```python
from build123d import *

# Parameters (mm, degrees)
SKETCH2_R               = 0.5
CUT_EXTRUDE1_DEPTH      = 4
CUT_EXTRUDE1_DEPTH_BACK = 4


with BuildPart() as part:
    # Sketch1 → Revolve1 (revolve)
    with BuildSketch(Plane.XY):
        with BuildLine():
            Line((0, 0), (0, 1.5))
            Line((0, 1.5), (0.5, 2))
            Line((0.5, 2), (39, 2))
            Line((39, 2), (39, 3))
            ThreePointArc((39, 3), (41.121320344, 2.121320344), (42, 0))
            Line((42, 0), (0, 0))
        make_face()
    revolve(axis=Axis((0, 0, 0), (1, 0, 0)))

    # Sketch2 → Cut-Extrude1 (cut, two sides)
    with BuildSketch(Plane.XY) as cut_extrude1_sk:
        with Locations((2, 0)):
            Circle(SKETCH2_R)
    extrude(amount=CUT_EXTRUDE1_DEPTH, mode=Mode.SUBTRACT)
    extrude(cut_extrude1_sk.sketch, amount=-CUT_EXTRUDE1_DEPTH_BACK, mode=Mode.SUBTRACT)


solid = part.part
```
Model file for the job. Use its own axes, mm. A direction names the side the tool comes from. Coordinates: 2 decimals unless noted, no trailing zeros. Loops run counter-clockwise (first coordinate to the right, second up) from the corner with the lowest first, then second, coordinate; pieces in that order, holes last. Notation, with made-up numbers: M 59.25,13 L 71.25,13 A20 ccw 71.25,22 Z; hole C 53,79 d7. An arc over 180 degrees is marked long. Use CSV: the item, a comma, the result in double quotes. Start each with the question number.
1. Band-saw the part on B-B, the plane x = 24. List the corners of the cut face in (y, z), then the cut area to 3 significant figures.
2. Band-saw the part on A-A, the plane y = 0. List the corners of the cut face in (x, z), then the cut area to 3 significant figures.
3. Flat gauge pins, fed straight in: pin 1 (1.5 mm diameter, centred on x = 27, z = -0.5, fed in from -Y); pin 2 (1 mm diameter, centred on x = 18, z = -1, fed in from -Y); pin 3 (1 mm diameter, centred on x = 17, y = 2, fed in from +Z). Where does each tip first touch, or does it go through?
4. Band-saw the part on D-D, the plane y = -2.6. List the corners of the cut face in (x, z), then the cut area to 3 significant figures.
5. Band-saw the part on C-C, the plane x = 2. List the corners of the cut face in (y, z).
6. Tool access for faces 1 (the cylindrical face through (20, 0, -2)), 2 (the flat face through (0, 0, 0)): list every direction of +Z, -Z, +X, -X, +Y, -Y with a clear straight run to the whole face (end or side of a thin tool).
7. Probe probe 1 along Y at (x, z) = (2, 0.6); probe 2 along X at (y, z) = (0, 0.45); probe 3 along Y at (x, z) = (2, -1.4). List the from-to ranges inside material, lowest first. Write a range as [from, to].
Entries:
1,outline,"C 0,0 d4"
1,area,"12.6 mm2"
2,outline,"M 0,-1.5 L 0.5,-2 L 1.5,-2 L 1.5,2 L 0.5,2 L 0,1.5 Z; M 2.5,-2 L 39,-2 L 39,-3 A3 ccw 39,3 L 39,2 L 2.5,2 Z"
2,area,"166 mm2"
3,pin 1,"stops at y = -2"
3,pin 2,"stops at y = -1.94"
3,pin 3,"stops at z = 1.32"
4,outline,"M 39,-1.5 A1.5 ccw 39,1.5 Z"
4,area,"3.52 mm2"
5,outline,"M -0.5,-1.94 L -0.5,1.94 A2 ccw Z; M 0.5,-1.94 A2 ccw 0.5,1.94 Z"
6,face 1,"-X"
6,face 2,"+Z, -Z, -X, +Y, -Y"
7,probe 1,"y = [-1.91, -0.5], [0.5, 1.91]"
7,probe 2,"x = [0, 1.5], [2.5, 41.97]"
7,probe 3,"y = [-1.43, -0.5], [0.5, 1.43]"
